Could you check a few things on this model? Use its own coordinates, in mm. A direction names the side the tool comes from. Round coordinates to 2 decimals unless told otherwise and drop trailing zeros. Loops run counter-clockwise (first coordinate to the right, second up) from the corner with the lowest first, then second, coordinate; pieces in that order, holes last. Notation, with made-up numbers: (64, -15.75) -> (90, -15.75) arc R25 cw to (90, 22.25) -> close; hole circle Ø3 at (37.5, 18.25). An arc over 180 degrees is marked (long way). One line per item, written item: value.
```python
from build123d import *

# Parameters (mm, degrees)
SKETCH2_R                                 = 1
BOSS_EXTRUDE3_DEPTH                       = 1.5875
DB15_PLUG_CUTAWAY_DEPTH                   = 55.106562968
CSK_FOR_4_FLAT_HEAD_MACHINE_SCREW_2_COUNT = 2
CSK_FOR_4_FLAT_HEAD_MACHINE_SCREW_2_PITCH = 51.65
CSK_FOR_4_FLAT_HEAD_MACHINE_SCREW_3_COUNT = 2
CSK_FOR_4_FLAT_HEAD_MACHINE_SCREW_3_PITCH = 81.65
CSK_FOR_4_FLAT_HEAD_MACHINE_SCREW_4_COUNT = 2
CSK_FOR_4_FLAT_HEAD_MACHINE_SCREW_4_PITCH = 96.614931558
SKETCH11_R                                = 1.7399
CUT_EXTRUDE1_DEPTH                        = 55.106562968


with BuildPart() as part:
    # Sketch2 → Boss-Extrude3 (new body)
    with BuildSketch(Plane(origin=(0, 0, 0), x_dir=(1, 0, 0), z_dir=(0, 1, 0))):
        with BuildLine():
            Line((-45, 25.825), (-45, -25.825))
            ThreePointArc((-45, -25.825), (-43.777170811, -28.777170811), (-40.825, -30))
            Line((-40.825, -30), (40.825, -30))
            ThreePointArc((40.825, -30), (43.777170811, -28.777170811), (45, -25.825))
            Line((45, -25.825), (45, 25.825))
            ThreePointArc((45, 25.825), (43.777170811, 28.777170811), (40.825, 30))
            Line((40.825, 30), (-40.825, 30))
            ThreePointArc((-40.825, 30), (-43.777170811, 28.777170811), (-45, 25.825))
        make_face()
        with Locations(Location((40.825, 25.825, 0), (0, 0, 270))):
            Circle(SKETCH2_R, mode=Mode.SUBTRACT)
        with Locations(Location((-40.825, 25.825, 0), (0, 0, 270))):
            Circle(SKETCH2_R, mode=Mode.SUBTRACT)
        with Locations(Location((-40.825, -25.825, 0), (0, 0, 270))):
            Circle(SKETCH2_R, mode=Mode.SUBTRACT)
        with Locations(Location((40.825, -25.825, 0), (0, 0, 270))):
            Circle(SKETCH2_R, mode=Mode.SUBTRACT)
    extrude(amount=BOSS_EXTRUDE3_DEPTH)

    # Sketch4 → DB15 Plug Cutaway (cut, through all)
    with BuildSketch(Plane.XZ):
        with BuildLine():
            Line((-13.835, 6.924614493), (-13.835, 11.090214492))
            ThreePointArc((-13.835, 11.090214492), (-12.684222543, 13.868437036), (-9.905999998, 15.019214492))
            Line((-9.905999998, 15.019214492), (9.905999999, 15.019214492))
            ThreePointArc((9.905999999, 15.019214492), (12.684222543, 13.868437035), (13.835, 11.090214492))
            Line((13.835, 11.090214492), (13.835, 6.924614492))
            ThreePointArc((13.835, 6.924614492), (12.684222543, 4.146391949), (9.906, 2.995614492))
            Line((9.906, 2.995614492), (-9.905999998, 2.995614492))
            ThreePointArc((-9.905999998, 2.995614492), (-12.684222543, 4.146391948), (-13.835, 6.924614493))
        make_face()
    extrude(amount=-DB15_PLUG_CUTAWAY_DEPTH, mode=Mode.SUBTRACT)

    # Sketch9 → CSK for #4 Flat Head Machine Screw (100)2 (revolve, cut)
    with BuildSketch(Plane(origin=(-40.825, 0, 25.825), x_dir=(0, 0, -1), z_dir=(1, 0, 0))):
        Polygon((0, 0), (0, 1.5875), (1.63195, 1.5875), (1.63195, 1.028358553), (2.8575, 0), align=None)
    csk_for_4_flat_head_machine_screw_100 = revolve(axis=Axis((-40.825, -6.35, 25.825), (0, 1, 0)), mode=Mode.SUBTRACT)

    # CSK for _4 Flat Head Machine Screw _ 2: CSK for #4 Flat Head Machine Screw (100)2 ×2
    with Locations(*[(0, 0, -i * CSK_FOR_4_FLAT_HEAD_MACHINE_SCREW_2_PITCH) for i in range(1, CSK_FOR_4_FLAT_HEAD_MACHINE_SCREW_2_COUNT)]):
        add(csk_for_4_flat_head_machine_screw_100, mode=Mode.SUBTRACT)

    # CSK for _4 Flat Head Machine Screw _ 3: CSK for #4 Flat Head Machine Screw (100)2 ×2
    with Locations(*[(i * CSK_FOR_4_FLAT_HEAD_MACHINE_SCREW_3_PITCH, 0, 0) for i in range(1, CSK_FOR_4_FLAT_HEAD_MACHINE_SCREW_3_COUNT)]):
        add(csk_for_4_flat_head_machine_screw_100, mode=Mode.SUBTRACT)

    # CSK for _4 Flat Head Machine Screw _ 4: CSK for #4 Flat Head Machine Screw (100)2 ×2
    with Locations(*[Vector(0.8451074661352507, 0, -0.5345964559202167) * (i * CSK_FOR_4_FLAT_HEAD_MACHINE_SCREW_4_PITCH) for i in range(1, CSK_FOR_4_FLAT_HEAD_MACHINE_SCREW_4_COUNT)]):
        add(csk_for_4_flat_head_machine_screw_100, mode=Mode.SUBTRACT)

    # Sketch11 → Cut-Extrude1 (cut, through all)
    with BuildSketch(Plane.XZ):
        with Locations(Location((-30.382, -0.009017528, 0), (0, 0, 270))):
            Circle(SKETCH11_R)
        with Locations(Location((30.382, -0.061487226, 0), (0, 0, 270))):
            Circle(SKETCH11_R)
    extrude(amount=-CUT_EXTRUDE1_DEPTH, mode=Mode.SUBTRACT)


solid = part.part
```
(1) We'd pull the mould along Z, two halves only. Please class faces 3 (the face through (42.418, 1.304, 26.179)), 4 (the face through (43.745, 0.783, 28.809)), 5 (the face through (-1, 1.588, 0)): +Z half, -Z half, draft (parallel to the pull), parting line (faces both ways), or undercut.
Results below:
face 3: undercut
face 4: +Z half
face 5: draft
(2) For pin 1 Ø4 at (x, z) = (30.38, -0.06) entering from -Y; pin 2 Ø2.5 at (x, z) = (40.825, 25.825) entering from -Y, each with a flat end and sliding along its axis, tell me the tip position at first contact or that it passes through.
Results below:
pin 1: stops at y = 0
pin 2: passes through
(3) Please list where these lines run through material, in increasing order: L1, parallel to Z at x = 41, y = 1.4; L2, parallel to X at y = 0.4, z = 24; L3, parallel to X at y = 1, z = 25.
Results below:
L1: z = -30 to -27.45, -24.2 to 24.2, 27.45 to 30
L2: x = -45 to -42.35, -39.3 to 39.3, 42.35 to 45
L3: x = -45 to -42.27, -39.38 to 39.38, 42.27 to 45
(4) On a 3-axis mill with a long thin cutter (end or side, diameter ignored), from which of +Z, -Z, +X, -X, +Y, -Y can I reach the whole of each face in a straight line? I mean faces 1 (the face through (12.65, 0.78, 13.9)), 2 (the face through (-1, 0, 0)). Say none if no direction works.
Results below:
face 1: +Y, -Y
face 2: +Z, -Z, +X, -X, -Y
(5) Imagine slicing it at A-A on z = 10. Write out the boundary of the cut face in (x, y) (1 decimal).
Results below:
outline: (-45, 0) -> (-13.8, 0) -> (-13.8, 1.6) -> (-45, 1.6) -> close; (13.8, 0) -> (45, 0) -> (45, 1.6) -> (13.8, 1.6) -> close
(6) Imagine slicing it at B-B on y = 0.3. Write out the boundary of the cut face in (x, z) (3 decimals).
Results below:
outline: (-45, -25.825) arc R4.175 ccw to (-40.825, -30) -> (40.825, -30) arc R4.175 ccw to (45, -25.825) -> (45, 25.825) arc R4.175 ccw to (40.825, 30) -> (-40.825, 30) arc R4.175 ccw to (-45, 25.825) -> close; hole circle Ø5 at (-40.825, -25.825); hole circle Ø5 at (-40.825, 25.825); hole circle Ø3.48 at (-30.382, -0.009); hole (-13.835, 6.925) arc R3.929 ccw to (-9.906, 2.996) -> (9.906, 2.996) arc R3.929 ccw to (13.835, 6.925) -> (13.835, 11.09) arc R3.929 ccw to (9.906, 15.019) -> (-9.906, 15.019) arc R3.929 ccw to (-13.835, 11.09) -> close; hole circle Ø3.48 at (30.382, -0.061); hole circle Ø5 at (40.825, -25.825); hole circle Ø5 at (40.825, 25.825)
